from build123d import *

# Parameters (mm, degrees)
SKETCH_1_R      = 12
SKETCH_1_R_2    = 1.25
EXTRUDE_1_DEPTH = 10


with BuildPart() as part:
    # Эскиз1 → Бобышка-Вытянуть1 (new body)
    with BuildSketch(Plane.XY):
        Polygon((-204.208503022, -30.605986098), (-138.208503022, -30.605986098), (-138.208503022, 1.294013902), (-145.008503022, 1.294013902), (-145.008503022, 0.094013902), (-147.208503022, 0.094013902), (-147.208503022, 1.294013902), (-148.708503022, 1.294013902), (-148.708503022, 4.394013902), (-147.208503022, 4.394013902), (-147.208503022, 5.594013902), (-145.008503022, 5.594013902), (-145.008503022, 4.394013902), (-138.208503022, 4.394013902), (-138.208503022, 204.394013902), (-140.975215975, 204.394013902), (-141.141859499, 214.392625303), (-151.141859499, 214.392625303), (-151.308503022, 204.394013902), (-169.658503022, 204.394013902), (-169.658503022, 197.594013902), (-168.458503022, 197.594013902), (-168.458503022, 195.394013902), (-169.658503022, 195.394013902), (-169.658503022, 193.894013902), (-172.758503022, 193.894013902), (-172.758503022, 195.394013902), (-173.958503022, 195.394013902), (-173.958503022, 197.594013902), (-172.758503022, 197.594013902), (-172.758503022, 204.394013902), (-191.108503022, 204.394013902), (-191.275146545, 214.392625303), (-201.275146545, 214.392625303), (-201.441790069, 204.394013902), (-204.208503022, 204.394013902), (-204.208503022, 184.394013902), (-214.207114422, 184.227370379), (-214.207114422, 174.227370379), (-204.208503022, 174.194013902), (-204.208503022, 155.844013902), (-197.408503022, 155.844013902), (-197.408503022, 157.044013902), (-195.208503022, 157.044013902), (-195.208503022, 155.844013902), (-193.708503022, 155.844013902), (-193.708503022, 152.744013902), (-195.208503022, 152.744013902), (-195.208503022, 151.544013902), (-197.408503022, 151.544013902), (-197.408503022, 152.744013902), (-204.208503022, 152.744013902), (-204.208503022, 134.394013902), (-214.207114422, 134.227370379), (-214.207114422, 124.227370379), (-204.208503022, 124.194013902), (-204.208503022, 49.594013902), (-214.207114422, 49.427370379), (-214.207114422, 39.427370379), (-204.208503022, 39.394013902), (-204.208503022, 21.044013902), (-197.408503022, 21.044013902), (-197.408503022, 22.244013902), (-195.208503022, 22.244013902), (-195.208503022, 21.044013902), (-193.708503022, 21.044013902), (-193.708503022, 17.944013902), (-195.208503022, 17.944013902), (-195.208503022, 16.744013902), (-197.408503022, 16.744013902), (-197.408503022, 17.944013902), (-204.208503022, 17.944013902), (-204.208503022, -0.405986098), (-214.207114422, -0.572629621), (-214.207114422, -10.572629621), (-204.208503022, -10.605986098), align=None)
        with Locations((-172.758503022, 171.470752074)):
            Circle(SKETCH_1_R, mode=Mode.SUBTRACT)
        with Locations((-172.758503022, 90.948356806)):
            Circle(SKETCH_1_R, mode=Mode.SUBTRACT)
        with Locations((-188.184986495, 60.909591185)):
            Circle(SKETCH_1_R_2, mode=Mode.SUBTRACT)
        with Locations((-193.156341495, 60.977449185)):
            Circle(SKETCH_1_R_2, mode=Mode.SUBTRACT)
        with Locations((-188.204296495, 123.199321185)):
            Circle(SKETCH_1_R_2, mode=Mode.SUBTRACT)
        with Locations((-193.175651495, 123.267179185)):
            Circle(SKETCH_1_R_2, mode=Mode.SUBTRACT)
        with BuildLine():
            Line((-186.351911088, 19.284478243), (-186.351911088, 34.284478243))
            ThreePointArc((-186.351911088, 34.284478243), (-187.851911088, 35.784478243), (-189.351911088, 34.284478243))
            Line((-189.351911088, 34.284478243), (-189.351911088, 19.284478243))
            ThreePointArc((-189.351911088, 19.284478243), (-187.851911088, 17.784478243), (-186.351911088, 19.284478243))
        make_face(mode=Mode.SUBTRACT)
        with BuildLine():
            Line((-155.351911088, 19.284478243), (-155.351911088, 34.284478243))
            ThreePointArc((-155.351911088, 34.284478243), (-156.851911088, 35.784478243), (-158.351911088, 34.284478243))
            Line((-158.351911088, 34.284478243), (-158.351911088, 19.284478243))
            ThreePointArc((-158.351911088, 19.284478243), (-156.851911088, 17.784478243), (-155.351911088, 19.284478243))
        make_face(mode=Mode.SUBTRACT)
        with BuildLine():
            Line((-155.351911088, -11.715521757), (-155.351911088, 3.284478243))
            ThreePointArc((-155.351911088, 3.284478243), (-156.851911088, 4.784478243), (-158.351911088, 3.284478243))
            Line((-158.351911088, 3.284478243), (-158.351911088, -11.715521757))
            ThreePointArc((-158.351911088, -11.715521757), (-156.851911088, -13.215521757), (-155.351911088, -11.715521757))
        make_face(mode=Mode.SUBTRACT)
        with BuildLine():
            Line((-186.351911088, -11.715521757), (-186.351911088, 3.284478243))
            ThreePointArc((-186.351911088, 3.284478243), (-187.851911088, 4.784478243), (-189.351911088, 3.284478243))
            Line((-189.351911088, 3.284478243), (-189.351911088, -11.715521757))
            ThreePointArc((-189.351911088, -11.715521757), (-187.851911088, -13.215521757), (-186.351911088, -11.715521757))
        make_face(mode=Mode.SUBTRACT)
        with BuildLine():
            Line((-183.601911088, 3.784478243), (-183.601911088, 18.784478243))
            ThreePointArc((-183.601911088, 18.784478243), (-172.351911088, 30.034478243), (-161.101911088, 18.784478243))
            Line((-161.101911088, 18.784478243), (-161.101911088, 3.784478243))
            ThreePointArc((-161.101911088, 3.784478243), (-172.351911088, -7.465521757), (-183.601911088, 3.784478243))
        make_face(mode=Mode.SUBTRACT)
    extrude(amount=EXTRUDE_1_DEPTH)


solid = part.part
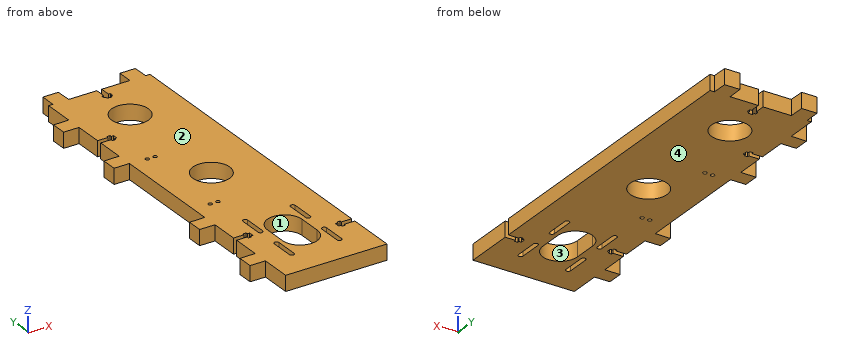
Input: part model. Units: mm. Frame: model coordinates. Face numbers are marked on the shaded views. A direction names the side the tool comes from. Give positions to 0.01 mm unless a question says otherwise; leave off trailing zeros. Write each loop counter-clockwise with the first axis right and the second up, starting at its lowest first coordinate (ties: lowest second). Pieces come first, ordered by that corner, then holes.
Q1. Set-up query: the marked faces 3 and 4. Return all of +Z, -Z, +X, -X, +Y, -Y with unobstructed straight access to the full face (end or side cutting, diameter ignored); none if empty.
Q2. Pull-direction query (Y, two-part tool) for the marked faces 1 and 2; classes: pulls with the +Y half, pulls with the -Y half, needs draft (parallel to the pull), parting line crosses it, or undercut.
Q3. Section C-C, the plane y = 163.5. Output: boundary loops of the cut face in (x, z).
Q4. Section A-A, the plane y = 96.5. Output: boundary loops of the cut face in (x, z), plus the area to 3 significant figures.
Q5. Section D-D, the plane z = 8. State how many separate pieces and enclosed holes the cut face has, plus the area to 3 significant figures.
Q6. Material intervals for probe 1 along X at (y, z) = (30.5, 4); probe 2 along Y at (x, z) = (-193, 2.25); probe 3 along Y at (x, z) = (-193.5, 1.5), sorted ascending.
Q7. First-contact query: P1, Ø2, axis at y = 88, z = 2, coming from the -X side; P2, Ø1, axis at x = -177.5, z = 4.5, coming from the +Y side; P3, Ø0.9, axis at y = 3, z = 4.5, coming from the +X side. Flat tips, straight axial feed; report the tip coordinate or a pass-through.
Q8. Section B-B, the plane x = -179. Output: boundary loops of the cut face in (y, z), plus the area to 3 significant figures.
Filled in:
1. face 3: +Z, -Z
1. face 4: -Z, +X, -X, +Y, -Y
2. face 1: undercut
2. face 2: needs draft
3. outline: (-204.21, 0) - (-181.73, 0) - (-181.73, 10) - (-204.21, 10) - close; (-163.79, 0) - (-138.21, 0) - (-138.21, 10) - (-163.79, 10) - close
4. outline: (-204.21, 0) - (-183.4, 0) - (-183.4, 10) - (-204.21, 10) - close; (-162.12, 0) - (-138.21, 0) - (-138.21, 10) - (-162.12, 10) - close
4. area: 447 mm2
5. separate pieces: 1
5. enclosed holes: 11
5. area: 14,100 mm2
6. probe 1: x = -204.21 to -189.35, -186.35 to -158.35, -155.35 to -138.21
6. probe 2: y = -30.61 to 59.74, 62.22 to 122.03, 124.5 to 214.39
6. probe 3: y = -30.61 to 59.78, 62.18 to 122.06, 124.47 to 214.39
7. P1: stops at x = -204.21
7. P2: stops at y = 204.39
7. P3: stops at x = -148.71
8. outline: (-30.61, 0) - (-5.29, 0) - (-5.29, 10) - (-30.61, 10) - close; (27.86, 0) - (80.7, 0) - (80.7, 10) - (27.86, 10) - close; (101.2, 0) - (161.22, 0) - (161.22, 10) - (101.2, 10) - close; (181.72, 0) - (204.39, 0) - (204.39, 10) - (181.72, 10) - close
8. area: 1,610 mm2
